Autodesk Inventor part; units mm, degrees
ref_plane "Płaszczyzna konstrukcyjna1" through (4.5, 1.15, 34.5) normal (1, 0, 0) x (0, 0, -1)
ref_plane "YZ Plane" through (0, 0, 0) normal (1, 0, 0) x (0, 1, 0)
ref_plane "XZ Plane" through (0, 0, 0) normal (0, 1, 0) x (-1, 0, 0)
sketch "Szkic2" plane through (0, 0, 0) normal (0, 0, 1) x (1, 0, 0)
  circle A0 centre (0, 0) radius 1.5
  circle A1 centre (8.3, 0) radius 1.5
  circle A2 centre (0, 0) radius 0.7
  circle A3 centre (8.3, 0) radius 0.7
  dimension "d0" = 3
  dimension "d1" = 8.3
  dimension "d2" = 3
  dimension "d3" = 1.4
  dimension "d4" = 1.4
sketch "Szkic3" plane through (0, 0, 0) normal (0, 0, 1) x (1, 0, 0)
  line L0 (0.9267, -1.15) -> (7.3733, -1.15)
  line L1 (7.3733, -1.15) -> (7.3733, 1.15)
  line L2 (7.3733, 1.15) -> (0.9267, 1.15)
  line L3 (0.9267, 1.15) -> (0.9267, -1.15)
  line L4 (0.9267, -1.15) -> (7.3733, 1.15) construction
  line L5 (7.3733, -1.15) -> (0.9267, 1.15) construction
  point P0 (0, 0)
  point P1 (4.15, 0)
  dimension "d5" = 4.15
  dimension "d6" = 2.3
extrude "Wyciągnięcie proste1" add sketch "Szkic2" along normal blind 45
extrude "Wyciągnięcie proste2" add sketch "Szkic3" along normal blind 45
sketch "Szkic4" plane through (0.9631, 1.15, 0) normal (0, 1, 0) x (1, 0, 0)
  line L0 (8.8369, 0) -> (8.8369, -45)
  line L1 (8.8369, 0) -> (8.8369, -3)
  line L2 (8.8369, -3) -> (0.5369, -3)
  line L3 (8.8369, -3) -> (5.8369, -3)
  line L4 (5.8369, -3) -> (5.8369, -4)
  line L5 (5.8369, -4) -> (8.8369, -4)
  line L6 (8.8369, -4) -> (8.8369, -3)
  line L7 (8.8369, -7.5) -> (5.8369, -7.5)
  line L8 (5.8369, -7.5) -> (5.8369, -12.5)
  line L9 (5.8369, -12.5) -> (8.8369, -12.5)
  line L10 (8.8369, -12.5) -> (8.8369, -7.5)
  line L11 (8.8369, -18.5) -> (5.8369, -18.5)
  line L12 (5.8369, -18.5) -> (5.8369, -23.5)
  line L13 (5.8369, -23.5) -> (8.8369, -23.5)
  line L14 (8.8369, -23.5) -> (8.8369, -18.5)
  line L15 (8.8369, -27.5) -> (5.8369, -27.5)
  line L16 (5.8369, -27.5) -> (5.8369, -34.5)
  line L17 (5.8369, -34.5) -> (8.8369, -34.5)
  line L18 (8.8369, -34.5) -> (8.8369, -27.5)
  line L19 (8.8369, -39) -> (5.8369, -39)
  line L20 (5.8369, -39) -> (5.8369, -45)
  line L21 (5.8369, -45) -> (8.8369, -45)
  line L22 (8.8369, -45) -> (8.8369, -39)
  line L23 (0, 0) -> (0, 0)
  line L24 (0, 0) -> (0, -45)
  line L25 (0, -45) -> (0, -45)
  line L26 (0, 0) -> (0, 0)
  line L27 (0, 0) -> (0, -45)
  line L28 (0, -45) -> (0, -45)
  line L29 (-2.4631, 0) -> (-2.4631, -45)
  line L30 (0, 0) -> (-2.4631, 0)
  line L31 (8.8369, 0) -> (6.3739, 0)
  line L32 (8.8369, 0) -> (0.5369, 0)
  line L33 (0.5369, 0) -> (0.5369, -3)
  line L34 (6.3739, 0) -> (0, 0)
  point P0 (-0.9631, 0)
  dimension "d11" = 3
  dimension "d12" = 5
  dimension "d13" = 3.5
  dimension "d14" = 1
  dimension "d15" = 5
  dimension "d16" = 6
  dimension "d17" = 7
  dimension "d18" = 4
  dimension "d19" = 4.5
  dimension "d20" = 6
  dimension "d21" = 3
  dimension "d22" = 3
  dimension "d23" = 3
  dimension "d24" = 3
  dimension "d26" = 3
  dimension "d27" = 3
extrude "Wyciągnięcie proste3" cut sketch "Szkic4" along normal mid plane 10
sketch "Szkic5" plane through (0.9631, 1.15, 45) normal (0, 1, 0) x (1, 0, 0)
  line L0 (6.3739, 6) -> (5.8369, 6) construction
  line L1 (0.5369, 41) -> (-2.4631, 41)
  line L2 (-2.4631, 41) -> (-2.4631, 36.5)
  line L3 (-2.4631, 36.5) -> (0.5369, 36.5)
  line L4 (0.5369, 36.5) -> (0.5369, 41)
  line L5 (0.6035, 32.5) -> (-2.4631, 32.5)
  line L6 (-2.4631, 32.5) -> (-2.4631, 25.5)
  line L7 (-2.4631, 25.5) -> (0.6035, 25.5)
  line L8 (0.6035, 25.5) -> (0.6035, 32.5)
  line L9 (0.5369, 21.5) -> (-2.4631, 21.5)
  line L10 (-2.4631, 21.5) -> (-2.4631, 16.5)
  line L11 (-2.4631, 16.5) -> (0.5369, 16.5)
  line L12 (0.5369, 16.5) -> (0.5369, 21.5)
  line L13 (0.5369, 10.5) -> (-2.4631, 10.5)
  line L14 (-2.4631, 10.5) -> (-2.4631, 5)
  line L15 (-2.4631, 5) -> (0.5369, 5)
  line L16 (0.5369, 5) -> (0.5369, 10.5)
  line L17 (0.5369, 2) -> (-2.4631, 2)
  line L18 (-2.4631, 2) -> (-2.4631, -1.3428)
  line L19 (-2.4631, -1.3428) -> (0.5369, -1.3428)
  line L20 (0.5369, -1.3428) -> (0.5369, 2)
  line L21 (6.3739, 17.5) -> (5.8369, 17.5)
  line L22 (5.8369, 17.5) -> (5.8369, 10.5)
  line L23 (5.8369, 10.5) -> (6.3739, 10.5)
  line L24 (6.3739, 6) -> (6.3739, 10.5)
  line L25 (6.3739, 6) -> (5.8369, 6)
  line L26 (5.8369, 6) -> (5.8369, 0)
  line L27 (0, 0) -> (5.8369, 0)
  line L28 (0, 45) -> (0, 0)
  line L29 (0, 45) -> (0.5369, 45)
  line L30 (0.5369, 45) -> (0.5369, 42)
  line L31 (0.5369, 42) -> (5.8369, 42)
  line L32 (5.8369, 42) -> (5.8369, 41)
  line L33 (5.8369, 41) -> (6.3739, 41)
  line L34 (6.3739, 37.5) -> (6.3739, 41)
  line L35 (6.3739, 37.5) -> (5.8369, 37.5)
  line L36 (5.8369, 37.5) -> (5.8369, 32.5)
  line L37 (5.8369, 32.5) -> (6.3739, 32.5)
  line L38 (6.3739, 26.5) -> (6.3739, 32.5)
  line L39 (6.3739, 26.5) -> (5.8369, 26.5)
  line L40 (5.8369, 26.5) -> (5.8369, 21.5)
  line L41 (5.8369, 21.5) -> (6.3739, 21.5)
  line L42 (6.3739, 17.5) -> (6.3739, 21.5)
  line L43 (5.8369, 12) -> (0.3369, 12)
  line L44 (0.3369, 12) -> (0.3369, 16)
  line L45 (0.3369, 16) -> (5.8369, 16)
  line L46 (5.8369, 16) -> (5.8369, 12)
  line L47 (-2.4631, 0) -> (0, 0)
  line L48 (0, 45) -> (-2.4631, 45)
  point P0 (-0.9631, 45)
  dimension "d32" = 3
  dimension "d33" = 5.5
  dimension "d34" = 4
  dimension "d35" = 1.5
  dimension "d78" = 5.5
  dimension "d79" = 6
  dimension "d80" = 5
  dimension "d81" = 4
  dimension "d82" = 7
  dimension "d83" = 4
  dimension "d84" = 4.5
  dimension "d85" = 2
  dimension "d86" = 4
extrude "Wyciągnięcie proste4" cut sketch "Szkic5" along normal mid plane 10 contours L4 L3 L28 L1 | L28 L3 L2 L1 | L28 L7 L6 L5 | L5 L8 L7 L28 | L28 L11 L10 L9 | L9 L12 L11 L28 | L28 L15 L14 L13 | L13 L16 L15 L28 | L28 L47 L18 L17 | L17 L20 L27 L28 | L27 L20 L19 L18 L47 | L43 L44 L45 L22
sketch "Szkic6" plane through (0, 0, 0) normal (0, 0, -1) x (-1, 0, 0)
  line L0 (-1, 1.5) -> (1.3193, 1.5) construction
  line L1 (-1.25, 1.5) -> (1.25, 1.5)
  line L2 (1.25, 1.5) -> (1.25, 4)
  line L3 (1.25, 4) -> (-1.25, 4)
  line L4 (-1.25, 4) -> (-1.25, 1.5)
  point P0 (0, 0)
  dimension "d36" = 1.5
  dimension "d37" = 2.5
  dimension "d38" = 2.5
  dimension "d39" = 1.25
extrude "Wyciągnięcie proste5" add sketch "Szkic6" against normal blind 43
chamfer "Faza1" distance 2 distance2 3.5 1 edges at (0, 4, 0) measured on face at (0, 3.1667, 0)
chamfer "Faza2" distance 2 distance2 3.5 1 edges at (0, 4, 43) measured on face at (0, 3.1667, 43)
sketch "Szkic7" plane through (-1.25, 1.5, 0) normal (-1, 0, 0) x (0, 0, 1)
  line L0 (39.5, 2.5) -> (43, 0.5)
  line L1 (3.5, 2.5) -> (39.5, 2.5)
  line L2 (0, 0.5) -> (3.5, 2.5)
  line L3 (0, 0) -> (0, 0.5)
  line L4 (0, 0) -> (43, 0)
  line L5 (43, 0.5) -> (43, 0)
  line L6 (0, 0) -> (4, 0)
  line L7 (0, -2.65) -> (0, 0)
  line L8 (0, -2.65) -> (4, -2.65)
  line L9 (4, -2.65) -> (4, 0)
  line L10 (4, 0) -> (4, -0.35)
  line L11 (4, -0.35) -> (0, -0.35)
  line L12 (0, 0) -> (0, -0.35)
  line L13 (8.5, 0) -> (12.5, 0)
  line L14 (8.5, 0) -> (8.5, -2.65)
  line L15 (8.5, -2.65) -> (12.5, -2.65)
  line L16 (12.5, -2.65) -> (12.5, 0)
  line L17 (12.5, 0) -> (12.5, -0.35)
  line L18 (12.5, -0.35) -> (8.5, -0.35)
  line L19 (8.5, -0.35) -> (8.5, 0)
  line L20 (19.5, 0) -> (23.5, 0)
  line L21 (19.5, 0) -> (19.5, -2.65)
  line L22 (19.5, -2.65) -> (23.5, -2.65)
  line L23 (23.5, -2.65) -> (23.5, 0)
  line L24 (23.5, 0) -> (23.5, -0.35)
  line L25 (23.5, -0.35) -> (19.5, -0.35)
  line L26 (19.5, -0.35) -> (19.5, 0)
  line L27 (28.5, 0) -> (34.5, 0)
  line L28 (28.5, 0) -> (28.5, -2.65)
  line L29 (28.5, -2.65) -> (34.5, -2.65)
  line L30 (34.5, -2.65) -> (34.5, 0)
  line L31 (34.5, 0) -> (34.5, -0.35)
  line L32 (34.5, -0.35) -> (28.5, -0.35)
  line L33 (28.5, -0.35) -> (28.5, 0)
  line L34 (40, 0) -> (43, 0)
  line L35 (40, 0) -> (40, -2.65)
  line L36 (40, -2.65) -> (43, -2.65)
  line L37 (43, -2.65) -> (43, 0)
  line L38 (43, 0) -> (43, -0.35)
  line L39 (43, -0.35) -> (40, -0.35)
  line L40 (40, -0.35) -> (40, 0)
  line L41 (40, -0.8) -> (43, -0.8)
  line L42 (43, -0.8) -> (40, -0.8)
  line L43 (40, -0.8) -> (40, 0)
  line L44 (40, 0) -> (43, 0)
  line L45 (43, 0) -> (43, -0.8)
  line L46 (34.5, -0.8) -> (28.5, -0.8)
  line L47 (28.5, -0.8) -> (28.5, 0)
  line L48 (28.5, 0) -> (34.5, 0)
  line L49 (34.5, 0) -> (34.5, -0.8)
  line L50 (23.5, -2.65) -> (23.5, -0.35)
  line L51 (23.5, -0.8) -> (19.5, -0.8)
  line L52 (19.5, -0.8) -> (19.5, 0)
  line L53 (19.5, 0) -> (23.5, 0)
  line L54 (23.5, 0) -> (23.5, -0.8)
  line L55 (12.5, -2.65) -> (12.5, -0.35)
  line L56 (12.5, -0.8) -> (8.5, -0.8)
  line L57 (8.5, -0.8) -> (8.5, 0)
  line L58 (8.5, 0) -> (12.5, 0)
  line L59 (12.5, 0) -> (12.5, -0.8)
  line L60 (0, 0) -> (43, 0)
  line L61 (4, -0.8) -> (0, -0.8)
  line L62 (0, -0.8) -> (0, 0)
  line L63 (0, 0) -> (4, 0)
  line L64 (4, 0) -> (4, -0.8)
extrude "Wyciągnięcie proste6" add sketch "Szkic7" against normal blind 2.5 contours L37 L39 L35 L4 | L37 L41 L35 L39 | L4 L9 L11 L7 | L30 L32 L28 L4 | L11 L9 L61 L7 | L30 L46 L28 L32 | L4 L16 L18 L14 | L23 L25 L21 L4 | L18 L16 L56 L14 | L23 L51 L21 L25
ref_plane "Płaszczyzna konstrukcyjna1" through (4.5, 1.15, 34.5) normal (1, 0, 0) x (0, 0, -1)
sketch "Szkic8" plane through (4.5, 1.15, 34.5) normal (1, 0, 0) x (0, 0, -1)
  line L0 (5.5, -2.3) -> (1.5, -2.3)
  line L1 (5.5, -2.3) -> (5.5, 0)
  line L2 (1.5, 0) -> (5.5, 0)
  line L3 (1.5, -2.3) -> (1.5, 0)
  line L4 (1.5, 0) -> (5.5, 0)
  line L5 (1.5, 0) -> (1.5, 1)
  line L6 (1.5, 1) -> (5.5, 1)
  line L7 (5.5, 1) -> (5.5, 0)
  line L8 (5.5, 0) -> (6.5, 0)
  line L9 (6, 0) -> (0, 0)
  line L10 (6.5, 0) -> (6.5, 2)
  line L11 (6.5, 2) -> (0.5, 2)
  line L12 (0.5, 2) -> (0.5, 0)
  line L13 (0, 0) -> (1.5, 0)
  line L14 (0.5, 0) -> (1.5, 0)
  point P0 (34.5, -1.15)
  dimension "d52" = 1
  dimension "d53" = 1
  dimension "d54" = 2
  dimension "d55" = 6
extrude "Wyciągnięcie proste7" add sketch "Szkic8" along normal blind 1 contours L7 L6 L5 L9 L12 L11 L10 L8
fillet "Zaokrąglenie1" radius 1 2 edges at (5, 3.15, 28) (5, 3.15, 34)
sketch "Szkic9" plane through (1.5, -1.15, 3) normal (0, -1, 0) x (1, 0, 0)
  line L0 (0, 5.5) -> (4.6429, 5.5)
  line L1 (4.6429, 5.5) -> (4.6429, 6.5)
  line L2 (4.6429, 6.5) -> (0, 6.5)
  line L3 (0, 6.5) -> (0, 5.5)
  line L4 (0, 20.5) -> (4.6429, 20.5)
  line L5 (4.6429, 20.5) -> (4.6429, 19.5)
  line L6 (4.6429, 19.5) -> (0, 19.5)
  line L7 (0, 19.5) -> (0, 20.5)
  line L8 (0, 0) -> (5.3, 0)
  point P0 (-1.5, -3)
  dimension "d74" = 13
  dimension "d75" = 5.5
  dimension "d76" = 1
  dimension "d77" = 1
extrude "Wyciągnięcie proste8" add sketch "Szkic9" along normal blind 5
chamfer "Faza3" distance 1 distance2 4 1 edges at (1.5, -6.15, 9) measured on face at (3.0476, -6.15, 9.1667)
chamfer "Faza4" distance 1 distance2 4 1 edges at (1.5, -6.15, 23) measured on face at (3.0476, -6.15, 23.1667)
chamfer "Faza5" distance 1 distance2 4 1 edges at (6.1429, -6.15, 23) measured on face at (3.7143, -6.15, 23.1667)
chamfer "Faza6" distance 1 distance2 4 1 edges at (6.1429, -6.15, 9) measured on face at (3.7143, -6.15, 9.1667)
fillet "Zaokrąglenie2" radius 1 4 edges at (2.5, -6.15, 9) (5.1429, -6.15, 9) (2.5, -6.15, 23) (5.1429, -6.15, 23)
sketch "Szkic10" plane through (1.5, -1.15, 23.5) normal (0, 0, 1) x (1, 0, 0)
  point P0 (-1.5, 1.15)
sketch "Szkic11" plane through (6.8, 1.15, 3) normal (0, 0, -1) x (-1, 0, 0)
  circle A0 centre (6.8, -1.15) radius 0.7
  circle A1 centre (-1.5, -1.15) radius 0.7
  dimension "d87" = 8.3
equation "\"d2\" = d0"
equation "\"d4\" = d3"
equation "\"d22\" = d21"
equation "\"d23\" = d22"
equation "\"d24\" = d23"
equation "\"d77\" = d76"
equation "\"dl_ogniwa\" = 9.073"
properties part number "ogniwo"
Check sheet for the modelled part. Datum: model origin and axes. Units: mm. A direction names the side the tool comes from. Coordinates: 2 decimals unless noted, no trailing zeros. Write each loop counter-clockwise with the first axis right and the second up, starting at its lowest first coordinate (ties: lowest second). Pieces come first, ordered by that corner, then holes.
Item 1: Mould release check, pull along Y, two halves, no side actions. Record for faces 1 (the face through (-0.7, 0, 2)), 2 (the face through (5.007, 2.849, 28.285)), 3 (the face through (8, 1, 23.5)): released by +Y, released by -Y, zero draft, split by the parting line, or undercut.
Numbers:
face 1: undercut
face 2: released by +Y
face 3: zero draft
Item 2: Cross-section at D-D on y = -3. Record the boundary of the cut face in (x, z).
Numbers:
outline: (1.71, 8.5) - (5.93, 8.5) - (5.93, 9.5) - (1.71, 9.5) - close; (1.71, 22.5) - (5.93, 22.5) - (5.93, 23.5) - (1.71, 23.5) - close
Item 3: Cross-section at C-C on z = 8. Record the boundary of the cut face in (x, y).
Numbers:
outline: (-1.25, 1.5) - (1.25, 1.5) - (1.25, 4) - (-1.25, 4) - close; (1.5, -1.15) - (6.8, -1.15) - (6.8, 1.15) - (1.5, 1.15) - close
Item 4: Access from +Z, -Z, +X, -X, +Y, -Y to the whole of each face (thin tool, end or side, straight path). Record for faces 4 (the face through (0, 1, 34.5)), 5 (the face through (4, -4, 23.5)), 6 (the face through (5, 3.15, 31)).
Numbers:
face 4: -X, -Y
face 5: +Z, -X, -Y
face 6: +Z, -Z, +X, +Y
Item 5: Cross-section at B-B on x = 8.3. Count the separate pieces of the cut face and the enclosed holes in it, then the cut area to 3 significant figures.
Numbers:
separate pieces: 8
enclosed holes: 0
area: 28.8 mm2
Item 6: Scan lines: probe 1 along Z at (x, y) = (2.75, -1.25); probe 2 along X at (y, z) = (0, 40.85); probe 3 along Y at (x, z) = (8.3, 38.15). Record each from-to range of solid material in increasing order.
Numbers:
probe 1: z = 8.5 to 9.5, 22.5 to 23.5
probe 2: x = -1.5 to -0.7, 0.7 to 6.8
probe 3: y = -1.5 to -0.7, 0.7 to 1.5
Item 7: Cross-section at A-A on z = 38. Record the boundary of the cut face in (x, y), then the cut area to 3 significant figures.
Numbers:
outline: (-1.25, 1.5) - (1.25, 1.5) - (1.25, 4) - (-1.25, 4) - close; (1.5, -1.15) - (7.34, -1.15) arc R1.5 ccw (long way) to (7.34, 1.15) - (1.5, 1.15) - close; hole circle Ø1.4 at (8.3, 0)
area: 24.3 mm2
Item 8: Depth check by flat-ended pin: pin 1 Ø3.5 at (x, y) = (9, -0.5) entering from +Z; pin 2 Ø1.5 at (x, y) = (0, 0) entering from -Z; pin 3 Ø1.8 at (x, y) = (0, 0) entering from +Z; pin 4 Ø1 at (x, z) = (4.5, 6) entering from -Y. Enter the tip coordinate at first touch or a pass-through.
Numbers:
pin 1: stops at z = 39
pin 2: stops at z = 0
pin 3: stops at z = 43
pin 4: stops at y = -1.15
